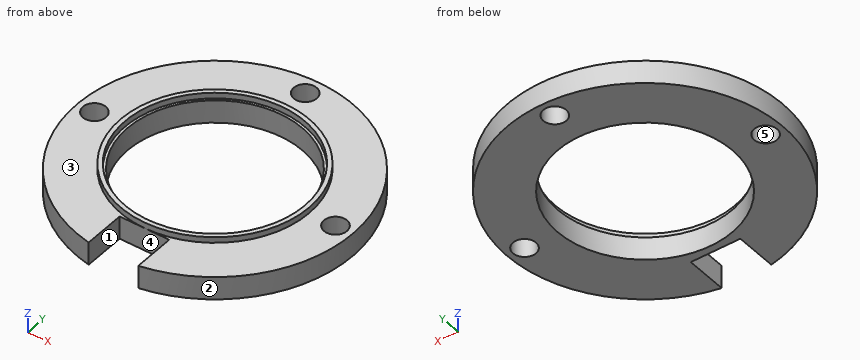
from build123d import *

# Parameters (mm, degrees)
SKETCH1_R           = 19.05
BOSS_EXTRUDE1_DEPTH = 3.175
SKETCH2_R           = 12.065
CUT_EXTRUDE1_DEPTH  = 4.175
SKETCH3_R           = 13.0175
SKETCH3_R_2         = 12.4175
BOSS_EXTRUDE2_DEPTH = 0.799999924
SKETCH4_W           = 6.858
SKETCH4_H           = 12.065
CUT_EXTRUDE2_DEPTH  = 4.175
SKETCH5_R           = 1.5875
CUT_EXTRUDE3_DEPTH  = 4.974999924


with BuildPart() as part:
    # Sketch1 → Boss-Extrude1 (new body)
    with BuildSketch(Plane.XY):
        Circle(SKETCH1_R)
    extrude(amount=BOSS_EXTRUDE1_DEPTH)

    # Sketch2 → Cut-Extrude1 (cut, through all)
    with BuildSketch(Plane.XY.offset(3.175)):
        Circle(SKETCH2_R)
    extrude(amount=-CUT_EXTRUDE1_DEPTH, mode=Mode.SUBTRACT)

    # Sketch3 → Boss-Extrude2 (add)
    with BuildSketch(Plane.XY.offset(3.175)):
        Circle(SKETCH3_R)
        Circle(SKETCH3_R_2, mode=Mode.SUBTRACT)
    extrude(amount=BOSS_EXTRUDE2_DEPTH)

    # Sketch4 → Cut-Extrude2 (cut, through all)
    with BuildSketch(Plane.XY.offset(3.175)):
        with Locations((0, -19.05)):
            Rectangle(SKETCH4_W, SKETCH4_H)
    extrude(amount=-CUT_EXTRUDE2_DEPTH, mode=Mode.SUBTRACT)

    # Sketch5 → Cut-Extrude3 (cut, through all)
    with BuildSketch(Plane(origin=(0, 0, 0), x_dir=(-1, 0, 0), z_dir=(0, 0, -1))):
        with Locations((-16.66875, 0)):
            Circle(SKETCH5_R)
        with Locations((0, 16.66875)):
            Circle(SKETCH5_R)
        with Locations((16.66875, 0)):
            Circle(SKETCH5_R)
    extrude(amount=-CUT_EXTRUDE3_DEPTH, mode=Mode.SUBTRACT)


solid = part.part
Work out the finished part from the listing and answer in its coordinate system (mm). Face numbers are marked on the shaded views. A direction names the side the tool comes from. Round coordinates to 2 decimals unless told otherwise and drop trailing zeros. Order: outer loops, then holes, each group sorted by start corner. A loop starts at its lowest first (then second) coordinate and runs counter-clockwise, first axis right, second up. Notation, with made-up numbers: M 62,-3 L 77,-3 A15 cw 77,14 Z; hole C 27.5,62 d11. An arc over 180 degrees is marked long. One line per item, written item: value.
Q1. Find section A-A on y = 0. Give the number of separate pieces and of enclosed holes in the cut face, then the cut area to 3 significant figures.
Derived:
separate pieces: 4
enclosed holes: 0
area: 25.2 mm²
Q2. Straight lines are drawn through the part: line 1 (Y direction, x = 0.5, z = 1.35); line 2 (Y direction, x = 0, z = 3.45); line 3 (X direction, y = -9, z = 1.55). For each, find the intervals that lie inside material, in ascending order.
Derived:
line 1: -13.02 to -12.05, 12.05 to 15.16, 18.18 to 19.04
line 2: -13.02 to -12.42, 12.42 to 13.02
line 3: -16.79 to -8.04, 8.04 to 16.79
Q3. Flat-ended cylindrical pins translate along their axes: pin 1 (1 mm diameter, centred on y = -1.5, z = 1, fed in from +X); pin 2 (1 mm diameter, centred on y = -9.5, z = 1, fed in from -X). Find the tip coordinate at first contact, or state that the pin passes through.
Derived:
pin 1: x = 19.02
pin 2: x = -16.79
Q4. For the marked faces 4 and 5, determine the directions among +Z, -Z, +X, -X, +Y, -Y from which every point of the face is accessible in a straight line to the end or side of a thin tool.
Derived:
face 4: +Z, -Z, -Y
face 5: +Z, -Z
Q5. Find section B-B on x = -5.5. Write down the section's boundary in (y, z) (3 decimals), then the cut area to 3 significant figures.
Derived:
outline: M -18.239,0 L -10.738,0 L -10.738,3.175 L -11.133,3.175 L -11.133,3.975 L -11.799,3.975 L -11.799,3.175 L -18.239,3.175 Z; M 10.738,0 L 18.239,0 L 18.239,3.175 L 11.799,3.175 L 11.799,3.975 L 11.133,3.975 L 11.133,3.175 L 10.738,3.175 Z
area: 48.7 mm²
Q6. Determine the mould class of the marked faces 1, 2 and 3 for opening direction X: released by +X, released by -X, zero draft, split by the parting line, or undercut.
Derived:
face 1: undercut
face 2: split by the parting line
face 3: zero draft
